Read the model definition and answer for the solid it produces. Units are mm, in the model's axes. A direction names the side the tool comes from. Coordinates: 2 decimals unless noted, no trailing zeros. Loops run counter-clockwise (first coordinate to the right, second up) from the corner with the lowest first, then second, coordinate; pieces in that order, holes last.
Q1. Section C-C (z = -4.5) is taken. Give the vertices of the cut face in (x, y).
Q2. Flat-ended cylindrical pins translate along their axes: P1, Ø1, axis at x = 26.5, y = -1, coming from the +Z side; P2, Ø0.8, axis at x = 44.5, y = 0, coming from the -Z side; P3, Ø1.5, axis at x = 18.5, z = 2.5, coming from the +Y side. Find the tip coordinate at first contact, or state that the pin passes through.
Q3. Which of the six approach directions +Z, -Z, +X, -X, +Y, -Y give full straight-line access (tool end or side, diameter ignored) to faces 1 (the face through (44.493, -1.776, -1.759)), 2 (the face through (44.5, -2.25, 0)), 3 (the face through (44.5, 0, -2.25)), 4 (the face through (44.493, 1.759, -1.776))?
Q4. Section A-A (x = 23) is taken. Give the vertices of the cut face in (y, z), then the cut area to 3 significant figures.
Q5. Section B-B (z = 4) is taken. Give the vertices of the cut face in (x, y), then the cut area to 3 significant figures.
Q6. Straight lines are drawn through the part: line 1 (Y direction, x = 2, z = 0.25); line 2 (X direction, y = 4.5, z = 1.5). For each, find the intervals that lie inside material, in ascending order.
from build123d import *

# Parameters (mm, degrees)
SKETCH1_R           = 5
BOSS_EXTRUDE1_DEPTH = 44
SKETCH2_R           = 2.5
BOSS_EXTRUDE2_DEPTH = 1
SKETCH3_OUTSIDE_W   = 21.434
SKETCH3_OUTSIDE_H   = 21.434
SKETCH3_OUTSIDE_W_2 = 4.5
SKETCH3_OUTSIDE_H_2 = 4.5
CUT_EXTRUDE1_DEPTH  = 1


with BuildPart() as part:
    # Sketch1 → Boss-Extrude1 (new body)
    with BuildSketch(Plane(origin=(0, 0, 0), x_dir=(0, 0, -1), z_dir=(1, 0, 0))):
        Circle(SKETCH1_R)
    extrude(amount=BOSS_EXTRUDE1_DEPTH)

    # Sketch2 → Boss-Extrude2 (add)
    with BuildSketch(Plane(origin=(44, 0, 0), x_dir=(0, 0, -1), z_dir=(1, 0, 0))):
        Circle(SKETCH2_R)
    extrude(amount=BOSS_EXTRUDE2_DEPTH)

    # Sketch3 outside → Cut-Extrude1 (cut)
    with BuildSketch(Plane(origin=(45, 0, 0), x_dir=(0, 0, -1), z_dir=(1, 0, 0))):
        Rectangle(SKETCH3_OUTSIDE_W, SKETCH3_OUTSIDE_H)
        Rectangle(SKETCH3_OUTSIDE_W_2, SKETCH3_OUTSIDE_H_2, mode=Mode.SUBTRACT)
    extrude(amount=-CUT_EXTRUDE1_DEPTH, mode=Mode.SUBTRACT)


solid = part.part
Numbers:
1. outline: (0, -2.18) - (44, -2.18) - (44, 2.18) - (0, 2.18) - close
2. P1: stops at z = 4.97
2. P2: stops at z = -2.25
2. P3: stops at y = 4.68
3. face 1: -Z, +X, -Y
3. face 2: +Z, -Z, +X, -Y
3. face 3: -Z, +X, +Y, -Y
3. face 4: -Z, +X, +Y
4. outline: circle Ø10 at (0, 0)
4. area: 78.5 mm2
5. outline: (0, -3) - (44, -3) - (44, 3) - (0, 3) - close
5. area: 264 mm2
6. line 1: y = -4.99 to 4.99
6. line 2: x = 0 to 44
